The listing builds one solid part. Answer for the finished solid, in the listing's coordinates (mm). Give positions to 0.01 mm unless a question says otherwise; leave off trailing zeros. Order: outer loops, then holes, each group sorted by start corner. A loop starts at its lowest first (then second) coordinate and runs counter-clockwise, first axis right, second up. Notation, with made-up numbers: (45.25, 52) - (60.25, 52) arc R10 cw to (60.25, 71) - close; hole circle Ø10 at (33, -17.75). An arc over 180 degrees is marked (long way). Use CSV: the item, a comma, the result in double quotes.
```python
from build123d import *

# Parameters (mm, degrees)
F0_R     = 2.5
F1_DEPTH = 2
F2_R     = 0.5
F3_SIZE  = 0.5
F4_SIZE  = 0.5
F5_R     = 0.5


with BuildPart() as f1:
    # F0 (on Front) → F1 (new body)
    with BuildSketch(Plane.XZ):
        with BuildLine():
            Line((7.1189217238, 7.4524198854), (-9.8810782762, 7.4524198854))
            ThreePointArc((-9.8810782762, 7.4524198854), (-15.3810782762, 1.9524198854), (-9.8810782762, -3.5475801146))
            Line((-9.8810782762, -3.5475801146), (7.1189217238, -3.5475801146))
            ThreePointArc((7.1189217238, -3.5475801146), (12.6189217238, 1.9524198854), (7.1189217238, 7.4524198854))
        make_face()
        with Locations((-9.8810782762, 1.9524198854)):
            Circle(F0_R, mode=Mode.SUBTRACT)
        with Locations((7.1189217238, 1.9524198854)):
            Circle(F0_R, mode=Mode.SUBTRACT)
    extrude(amount=F1_DEPTH)

    # F2
    f2_edges = [f1.edges().sort_by_distance(p)[0] for p in [
        (-1.381078, -2, 7.45242),
    ]]
    fillet(f2_edges, radius=F2_R)

    # F3
    f3_edges = [f1.edges().sort_by_distance(p)[0] for p in [
        (-12.381078, -2, 1.95242),
        (4.618922, -2, 1.95242),
    ]]
    chamfer(f3_edges, length=F3_SIZE)

    # F4
    f4_edges = [f1.edges().sort_by_distance(p)[0] for p in [
        (-12.381078, 0, 1.95242),
        (-1.381078, 0, 7.45242),
        (-15.381078, 0, 1.95242),
        (-1.381078, 0, -3.54758),
        (12.618922, 0, 1.95242),
        (4.618922, 0, 1.95242),
    ]]
    chamfer(f4_edges, length=F4_SIZE)

    # F5
    f5_edges = [f1.edges().sort_by_distance(p)[0] for p in [
        (-1.381078, -0.5, -3.54758),
    ]]
    fillet(f5_edges, radius=F5_R)


solid = f1.part
```
Item 1: The part is cut by section A-A (x = 3.25). Give the vertices of the cut face in (y, z).
Taken from the geometry:
outline,"(-2, -3.05) arc R0.5 ccw to (-1.5, -3.55) - (-0.71, -3.55) arc R0.5 ccw to (-0.35, -3.4) - (0, -3.05) - (0, 6.95) - (-0.35, 7.31) arc R0.5 ccw to (-0.71, 7.45) - (-1.5, 7.45) arc R0.5 ccw to (-2, 6.95) - close"
Item 2: The mould has two halves that part along X. Classify faces 1 (the face through (-2, 0, 2)), 2 (the face through (4.62, -0.99, 2.06)), 3 (the face through (12.253, -0.135, 1.84)): +X half, -X half, draft (parallel to the pull), parting line (faces both ways), or undercut.
Taken from the geometry:
face 1,"draft"
face 2,"undercut"
face 3,"+X half"
Item 3: The part is cut by section B-B (y = -1.25). Give the vertices of the cut face in (x, z), and give its area (3 significant figures).
Taken from the geometry:
outline,"(-9.88, -3.55) - (7.12, -3.55) arc R5.5 ccw to (7.12, 7.45) - (-9.88, 7.45) arc R5.5 ccw to start; hole circle Ø5 at (-9.88, 1.95); hole circle Ø5 at (7.12, 1.95)"
area,"243 mm^2"
Item 4: Find the intervals of material crossed by line 1 along Z through (x, y) = (-9.75, -0.75); line 2 along X through (y, z) = (-0.8, 1.75); line 3 along X through (y, z) = (-1.35, 3.75), in increasing order.
Taken from the geometry:
line 1,"-3.55 to -0.54, 4.45 to 7.45"
line 2,"-15.38 to -12.37, -7.39 to 4.63, 9.61 to 12.62"
line 3,"-15.08 to -11.62, -8.14 to 5.38, 8.86 to 12.32"
Item 5: The part is cut by section C-C (z = 0.5). Count the separate pieces of the cut face and the enclosed holes in it, and give its area (3 significant figures).
Taken from the geometry:
separate pieces,"3"
enclosed holes,"0"
area,"37.4 mm^2"
